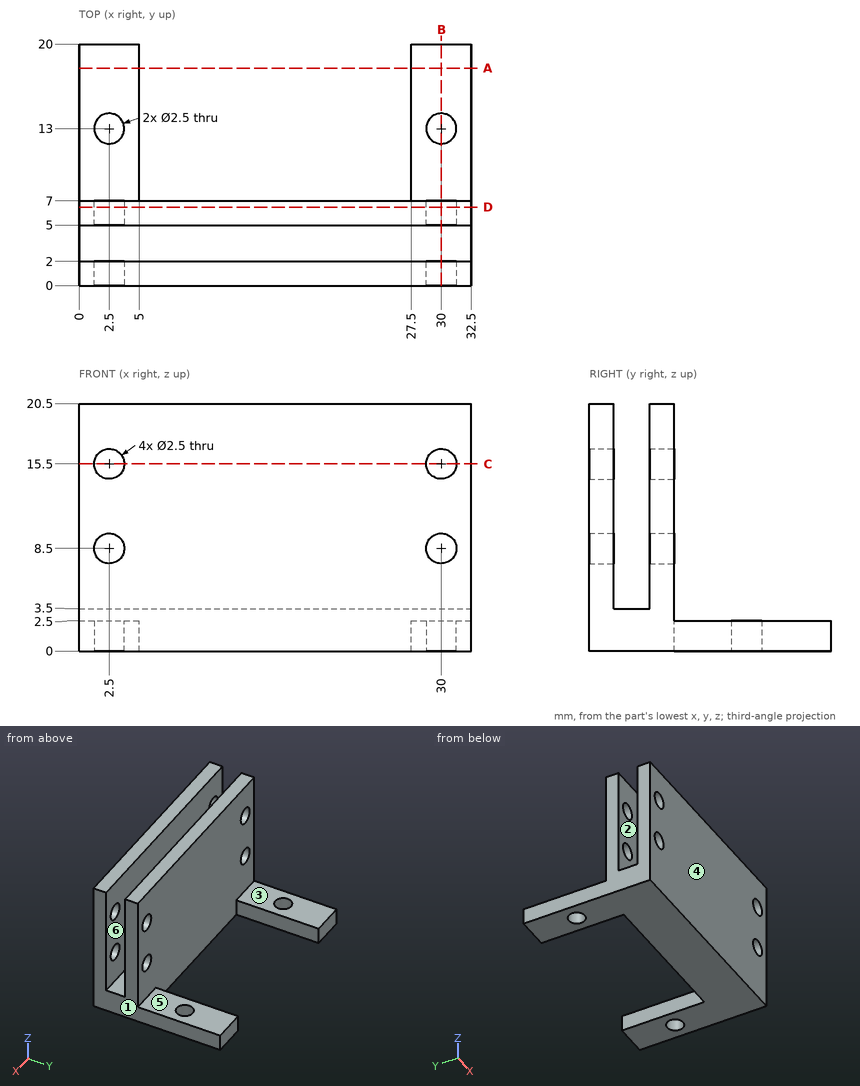
For this review, use the dimensioned drawing (mm, ordinates from the lowest corner) and the shaded views. A direction names the side the tool comes from. Coordinates: 2 decimals unless noted, no trailing zeros. Loops run counter-clockwise (first coordinate to the right, second up) from the corner with the lowest first, then second, coordinate; pieces in that order, holes last. Notation, with made-up numbers: (79, 44.5) -> (108, 44.5) arc R26 cw to (108, 64.5) -> close; hole circle Ø6 at (20, 65). An arc over 180 degrees is marked (long way). Write each question's results on one line, items separated by ' | '.
Q1. For pin 1 Ø3 at (x, z) = (30, 8.5) entering from +Y; pin 2 Ø1.5 at (x, y) = (16.5, 4) entering from +Z; pin 3 Ø2 at (x, z) = (2.5, 15.5) entering from +Y; pin 4 Ø4 at (x, y) = (1.5, 13.5) entering from +Z, all flat-tipped, find the tip position at first contact; note any pin that passes through.
Taken from the geometry:
pin 1: y = 7 | pin 2: z = 3.5 | pin 3: through | pin 4: z = 2.5
Q2. To check wall thickness, follow line 1 along Z through (x, y) = (2.5, 1.15); line 2 along X through (y, z) = (6.15, 8.5); line 3 along Y through (x, z) = (27, 5). State the ranges of each line that lie inside material, in increasing order. Write a range as [from, to].
Taken from the geometry:
line 1: [0, 7.25], [9.75, 14.25], [16.75, 20.5] | line 2: [0, 1.25], [3.75, 28.75], [31.25, 32.5] | line 3: [0, 2], [5, 7]
Q3. Add section A-A, the plane y = 18. State the section outline as (x, z) points, then the cut area to 3 significant figures.
Taken from the geometry:
outline: (0, 0) -> (5, 0) -> (5, 2.5) -> (0, 2.5) -> close; (27.5, 0) -> (32.5, 0) -> (32.5, 2.5) -> (27.5, 2.5) -> close | area: 25.0 mm²
Q4. Mouldability with a two-part tool opening along Y and no side actions: class the marked faces 4, 5 and 6 as +Y half, -Y half, draft (parallel to the pull), parting line (faces both ways), or undercut.
Taken from the geometry:
face 4: -Y half | face 5: draft | face 6: undercut
Q5. Add section C-C, the plane z = 15.5. State the section outline as (x, y) points, then the cut area to 3 significant figures.
Taken from the geometry:
outline: (0, 0) -> (1.25, 0) -> (1.25, 2) -> (0, 2) -> close; (0, 5) -> (1.25, 5) -> (1.25, 7) -> (0, 7) -> close; (3.75, 0) -> (28.75, 0) -> (28.75, 2) -> (3.75, 2) -> close; (3.75, 5) -> (28.75, 5) -> (28.75, 7) -> (3.75, 7) -> close; (31.25, 0) -> (32.5, 0) -> (32.5, 2) -> (31.25, 2) -> close; (31.25, 5) -> (32.5, 5) -> (32.5, 7) -> (31.25, 7) -> close | area: 110 mm²
Q6. Add section B-B, the plane x = 30. Count the separate pieces of the cut face and the enclosed holes in it, then the cut area to 4 significant figures.
Taken from the geometry:
separate pieces: 6 | enclosed holes: 0 | area: 98.75 mm²
Q7. Machinability: for the marked faces 1, 2 and 3, which of the approach directions +Z, -Z, +X, -X, +Y, -Y give a long, thin tool a straight path to every point of the face, cutting with its end or side? Answer none if there is none.
Taken from the geometry:
face 1: +Z, -Z, +X, +Y, -Y | face 2: +Z, +X, -X | face 3: +Z, +X, -X, +Y
Q8. Add section D-D, the plane y = 6.5. State the section outline as (x, z) points.
Taken from the geometry:
outline: (0, 0) -> (32.5, 0) -> (32.5, 20.5) -> (0, 20.5) -> close; hole circle Ø2.5 at (2.5, 8.5); hole circle Ø2.5 at (2.5, 15.5); hole circle Ø2.5 at (30, 8.5); hole circle Ø2.5 at (30, 15.5)
